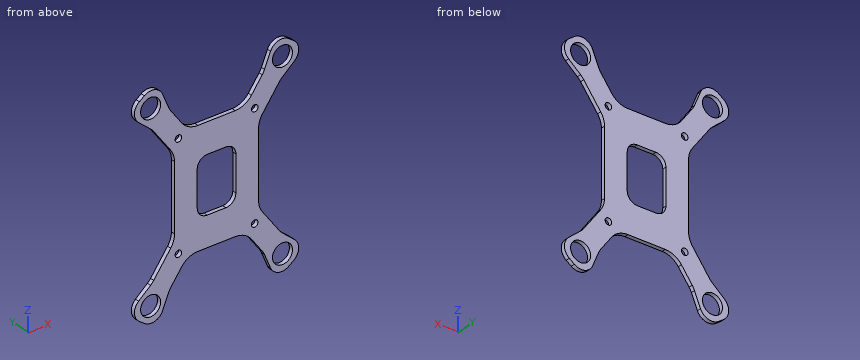
from build123d import *

# Parameters (mm, degrees)
SKETCH_1_W             = 42
SKETCH_1_H             = 57.75
EXTRUDE_1_DEPTH        = 2
EXTRUDE_2_DEPTH        = 2
SKETCH_8_W             = 19.31744652
SKETCH_8_H             = 27.856514232
CUT_EXTRUDE_4_DEPTH    = 9
FILLET_4_R             = 5
SKETCH_5_R             = 5
CUT_EXTRUDE_6_DEPTH    = 10
EXTRUDE_3_DEPTH        = 2
FILLET_5_R             = 10
FILLET_6_R             = 6
FILLET_5_OF_MIRROR_1_R = 10
FILLET_6_OF_MIRROR_1_R = 6
MIRROR_2_OUTLINE_R     = 5
MIRROR_2_DEPTH         = 2
SKETCH_3_R             = 1.65
CUT_EXTRUDE_1_DEPTH    = 68.321095486
FILLET_7_R             = 10


# Read off the part's stored shape, not the designer's step: 镜向2
with BuildPart() as part:
    # 草图1 → 凸台-拉伸1 (new body)
    with BuildSketch(Plane(origin=(0, 0, 0), x_dir=(1, 0, 0), z_dir=(0, 1, 0))):
        Rectangle(SKETCH_1_W, SKETCH_1_H)
    extrude(amount=EXTRUDE_1_DEPTH)

    # 草图2 → 凸台-拉伸2 (add)
    with BuildSketch(Plane(origin=(0, 2, 0), x_dir=(1, 0, 0), z_dir=(0, 1, 0))):
        Polygon((-12.413267133, 26.094069469), (-21, 19.849172839), (-41.586009419, 48.154935789), (-32.999276552, 54.39983242), align=None)
    extrude_2 = extrude(amount=-EXTRUDE_2_DEPTH)

    # 草图8 → 切除-拉伸4 (cut)
    with BuildSketch(Plane(origin=(0, 2, 0), x_dir=(1, 0, 0), z_dir=(0, 1, 0))):
        Rectangle(SKETCH_8_W, SKETCH_8_H)
    extrude(amount=-CUT_EXTRUDE_4_DEPTH, mode=Mode.SUBTRACT)

    # 圆角4
    fillet_4_edges = [part.edges().sort_by_distance(p)[0] for p in [
        (-9.65872326, 1, 13.928257116),
        (-9.65872326, 1, -13.928257116),
        (9.65872326, 1, -13.928257116),
        (9.65872326, 1, 13.928257116),
    ]]
    fillet(fillet_4_edges, radius=FILLET_4_R)

    # 草图5 → 切除-拉伸6 (cut)
    with BuildSketch(Plane(origin=(0, 2, 0), x_dir=(1, 0, 0), z_dir=(0, 1, 0))):
        with Locations(Location((-32.934365155, 45.284752088, 0), (0, 0, 270))):
            Circle(SKETCH_5_R)
    cut_extrude_6 = extrude(amount=-CUT_EXTRUDE_6_DEPTH, mode=Mode.SUBTRACT)

    # 草图9 → 凸台-拉伸3 (add)
    with BuildSketch(Plane(origin=(0, 2, 0), x_dir=(1, 0, 0), z_dir=(0, 1, 0))):
        Polygon((-32.07479568, 35.077016899), (-44.691673686, 45.896270868), (-41.586009419, 48.154935789), align=None)
        Polygon((-23.488062813, 41.321913529), (-29.893612284, 56.658497342), (-32.999276552, 54.39983242), align=None)
    extrude_3 = extrude(amount=-EXTRUDE_3_DEPTH)

    # 圆角5
    fillet_5_edges = [part.edges().sort_by_distance(p)[0] for p in [
        (-32.07479568, 1, -35.077016899),
        (-23.488062813, 1, -41.321913529),
    ]]
    fillet(fillet_5_edges, radius=FILLET_5_R)

    # 圆角6
    fillet_6_edges = [part.edges().sort_by_distance(p)[0] for p in [
        (-44.691673686, 1, -45.896270868),
        (-29.893612284, 1, -56.658497342),
    ]]
    fillet(fillet_6_edges, radius=FILLET_6_R)

    # 镜向1: 凸台-拉伸2, 切除-拉伸6, 凸台-拉伸3 across plane
    add(extrude_2.mirror(Plane(origin=(0, 0, 0), x_dir=(0, 0, 1), z_dir=(1, 0, 0))))
    add(cut_extrude_6.mirror(Plane(origin=(0, 0, 0), x_dir=(0, 0, 1), z_dir=(1, 0, 0))), mode=Mode.SUBTRACT)
    add(extrude_3.mirror(Plane(origin=(0, 0, 0), x_dir=(0, 0, 1), z_dir=(1, 0, 0))))

    # 圆角5 of 镜向1
    fillet_5_of_mirror_1_edges = [part.edges().sort_by_distance(p)[0] for p in [
        (32.07479568, 1, -35.077016899),
        (23.488062813, 1, -41.321913529),
    ]]
    fillet(fillet_5_of_mirror_1_edges, radius=FILLET_5_OF_MIRROR_1_R)

    # 圆角6 of 镜向1
    fillet_6_of_mirror_1_edges = [part.edges().sort_by_distance(p)[0] for p in [
        (44.691673686, 1, -45.896270868),
        (29.893612284, 1, -56.658497342),
    ]]
    fillet(fillet_6_of_mirror_1_edges, radius=FILLET_6_OF_MIRROR_1_R)

    # 镜向2 outline → 镜向2 (add)
    # profile 1 of 2: a face of its own
    with BuildSketch(Plane(origin=(0, 0, 0), x_dir=(1, 0, 0), z_dir=(0, 1, 0))):
        with BuildLine():
            Line((21, -28.875), (14.435762065, -28.875))
            Line((14.435762065, -28.875), (22.799263539, -40.374814527))
            ThreePointArc((22.799263539, -40.374814527), (23.428494894, -41.355407098), (23.939399044, -42.402532133))
            Line((23.939399044, -42.402532133), (26.967769787, -49.653254641))
            ThreePointArc((26.967769787, -49.653254641), (30.885501706, -53.118362872), (36.033297782, -52.193271525))
            Line((36.033297782, -52.193271525), (38.551988188, -50.361496684))
            ThreePointArc((38.551988188, -50.361496684), (41.018152801, -45.749162076), (38.928702373, -40.954394579))
            Line((38.928702373, -40.954394579), (32.963783297, -35.839343585))
            ThreePointArc((32.963783297, -35.839343585), (32.12501319, -35.030666519), (31.385996405, -34.129917896))
            Line((31.385996405, -34.129917896), (21, -19.849172839))
            Line((21, -19.849172839), (21, -28.875))
        make_face()
        with Locations((32.934365155, -45.284752088)):
            Circle(MIRROR_2_OUTLINE_R, mode=Mode.SUBTRACT)
    # profile 2 of 2: a face of its own
    with BuildSketch(Plane(origin=(0, 0, 0), x_dir=(1, 0, 0), z_dir=(0, 1, 0))):
        with BuildLine():
            Line((-22.799263539, -40.374814527), (-14.435762065, -28.875))
            Line((-14.435762065, -28.875), (-21, -28.875))
            Line((-21, -28.875), (-21, -19.849172839))
            Line((-21, -19.849172839), (-31.385996405, -34.129917896))
            ThreePointArc((-31.385996405, -34.129917896), (-32.12501319, -35.030666519), (-32.963783297, -35.839343585))
            Line((-32.963783297, -35.839343585), (-38.928702373, -40.954394579))
            ThreePointArc((-38.928702373, -40.954394579), (-41.018152801, -45.749162076), (-38.551988188, -50.361496684))
            Line((-38.551988188, -50.361496684), (-36.033297782, -52.193271525))
            ThreePointArc((-36.033297782, -52.193271525), (-30.885501706, -53.118362872), (-26.967769787, -49.653254641))
            Line((-26.967769787, -49.653254641), (-23.939399044, -42.402532133))
            ThreePointArc((-23.939399044, -42.402532133), (-23.428494894, -41.355407098), (-22.799263539, -40.374814527))
        make_face()
        with Locations((-32.934365155, -45.284752088)):
            Circle(MIRROR_2_OUTLINE_R, mode=Mode.SUBTRACT)
    extrude(amount=MIRROR_2_DEPTH)

    # 草图3 → 切除-拉伸1 (cut, through all)
    with BuildSketch(Plane(origin=(0, 2, 0), x_dir=(1, 0, 0), z_dir=(0, 1, 0))):
        with Locations(Location((19.05, 26.415, 0), (0, 0, 270))):
            Circle(SKETCH_3_R)
        with Locations(Location((19.05, -26.415, 0), (0, 0, 90))):
            Circle(SKETCH_3_R)
        with Locations(Location((-19.05, -26.415, 0), (0, 0, 270))):
            Circle(SKETCH_3_R)
        with Locations(Location((-19.05, 26.415, 0), (0, 0, 90))):
            Circle(SKETCH_3_R)
    extrude(amount=-CUT_EXTRUDE_1_DEPTH, mode=Mode.SUBTRACT)

    # 圆角7
    fillet_7_edges = [part.edges().sort_by_distance(p)[0] for p in [
        (14.435762065, 1, -28.875),
        (21, 1, -19.849172839),
        (-21, 1, -19.849172839),
        (-14.435762065, 1, -28.875),
        (21, 1, 19.849172839),
        (14.435762065, 1, 28.875),
        (-14.435762065, 1, 28.875),
        (-21, 1, 19.849172839),
    ]]
    fillet(fillet_7_edges, radius=FILLET_7_R)


solid = part.part
Verification items for the finished model (mm, model axes). Coordinates: 2 decimals unless noted, no trailing zeros. Order: outer loops, then holes, each group sorted by start corner. A loop starts at its lowest first (then second) coordinate and runs counter-clockwise, first axis right, second up. Notation, with made-up numbers: M 78,-38.75 L 110,-38.75 A20 cw 110,-5.75 Z; hole C 5,36.5 d2. An arc over 180 degrees is marked long. Write each question's results on one line, items separated by ' | '.
1) Gauge pin test, flat ends, axial feed: pin 1 Ø0.6 at (y, z) = (1.5, 3) entering from +X; pin 2 Ø0.6 at (x, y) = (-4.5, 1) entering from -Z (3 decimals); pin 3 Ø1 at (y, z) = (1.5, 4) entering from -X. Record the tip position at first contact, or that the pin passes through.
Solved:
pin 1: stops at x = 21 | pin 2: stops at z = -28.875 | pin 3: stops at x = -21
2) Section check C-C on y = 0.65. Give the number of separate pieces and of enclosed holes in the cut face, plus the area to 3 significant figures.
Solved:
separate pieces: 1 | enclosed holes: 9 | area: 3,020 mm²
3) Section check A-A on x = 6. Record the cut outline in (y, z) (3 decimals), plus the area to 3 significant figures.
Solved:
outline: M 0,-28.875 L 2,-28.875 L 2,-13.745 L 0,-13.745 Z; M 0,13.745 L 2,13.745 L 2,28.875 L 0,28.875 Z | area: 60.5 mm²
4) Section check B-B on x = -19.05. Record the cut outline in (y, z) (3 decimals).
Solved:
outline: M 0,-35.22 L 2,-35.22 L 2,-28.065 L 0,-28.065 Z; M 0,-24.765 L 2,-24.765 L 2,24.765 L 0,24.765 Z; M 0,28.065 L 2,28.065 L 2,35.22 L 0,35.22 Z
5) Scan lines: line 1 along Z through (x, y) = (19, 0.2); line 2 along X through (y, z) = (1.45, -27); line 3 along Z through (x, y) = (4, 1.5) (3 decimals). Record each from-to range of solid material in increasing order. Write a range as [from, to].
Solved:
line 1: z = [-35.15, -28.06], [-24.77, 24.77], [28.06, 35.15] | line 2: x = [-26.2, -20.59], [-17.51, 17.51], [20.59, 26.2] | line 3: z = [-28.875, -13.928], [13.928, 28.875]
